```python
from build123d import *

# Parameters (mm, degrees)
SKETCH_1_W          = 200
SKETCH_1_H          = 200
EXTRUDE_1_DEPTH     = 1.5
SKETCH_2_R          = 2.5
CUT_EXTRUDE_1_DEPTH = 1.5


with BuildPart() as part:
    # 草图1 → 凸台-拉伸1 (new body)
    with BuildSketch(Plane.XY):
        Rectangle(SKETCH_1_W, SKETCH_1_H)
    extrude(amount=EXTRUDE_1_DEPTH)

    # 草图2 → 切除-拉伸1 (cut)
    with BuildSketch(Plane.XY.offset(1.5)):
        with Locations((-35, -82)):
            Circle(SKETCH_2_R)
        with Locations((-35, -59)):
            Circle(SKETCH_2_R)
        with Locations(Location((35, -82, 0), (0, 0, 180))):
            Circle(SKETCH_2_R)
        with Locations(Location((35, -59, 0), (0, 0, 180))):
            Circle(SKETCH_2_R)
    extrude(amount=-CUT_EXTRUDE_1_DEPTH, mode=Mode.SUBTRACT)


solid = part.part
```
Could you check a few things on this model? Use its own coordinates, in mm. Round coordinates to 2 decimals unless told otherwise and drop trailing zeros. Loops run counter-clockwise (first coordinate to the right, second up) from the corner with the lowest first, then second, coordinate; pieces in that order, holes last. Notation, with made-up numbers: M 40.25,-27.5 L 90.25,-27.5 A18 ccw 90.25,5.5 Z; hole C 64,-40 d6. An arc over 180 degrees is marked long. Put each result on its own line as item: value.
Q1. Imagine slicing it at B-B (x = -35). Write out the boundary of the cut face in (y, z), then the cut area to 3 significant figures.
Check result:
outline: M -100,0 L -84.5,0 L -84.5,1.5 L -100,1.5 Z; M -79.5,0 L -61.5,0 L -61.5,1.5 L -79.5,1.5 Z; M -56.5,0 L 100,0 L 100,1.5 L -56.5,1.5 Z
area: 285 mm2
Q2. Imagine slicing it at A-A (y = -59). Write out the boundary of the cut face in (x, z).
Check result:
outline: M -100,0 L -37.5,0 L -37.5,1.5 L -100,1.5 Z; M -32.5,0 L 32.5,0 L 32.5,1.5 L -32.5,1.5 Z; M 37.5,0 L 100,0 L 100,1.5 L 37.5,1.5 Z
Q3. I need wall thicknesses on probe 1 along Y at (x, z) = (35, 0.55); probe 2 along Y at (x, z) = (-36, 0.8). Which ranges of each line are inside material? Lowest first, please.
Check result:
probe 1: -100 to -84.5, -79.5 to -61.5, -56.5 to 100
probe 2: -100 to -84.29, -79.71 to -61.29, -56.71 to 100
Q4. Thinking about a two-plate mould opening in X: for faces 1 (the face through (32.69, -81.04, 0.76)), 2 (the face through (-1, 1, 1.5)), which applies, released by +X, released by -X, zero draft, split by the parting line, or undercut?
Check result:
face 1: undercut
face 2: zero draft
Q5. For pin 1 (2 mm diameter, centred on x = 46.5, y = -39.5, fed in from -Z), with a flat end and sliding along its axis, tell me the tip position at first contact or that it passes through.
Check result:
pin 1: z = 0
